Input: part model. Units: mm. Frame: model coordinates. Face numbers are marked on the shaded views. A direction names the side the tool comes from. Round coordinates to 2 decimals unless told otherwise and drop trailing zeros. Order: outer loops, then holes, each group sorted by start corner. A loop starts at its lowest first (then second) coordinate and runs counter-clockwise, first axis right, second up. Notation, with made-up numbers: (86.5, 65.25) -> (111.5, 65.25) arc R31 cw to (111.5, 94.25) -> close; hole circle Ø5 at (-17.5, 79.5). An arc over 180 degrees is marked (long way). Use a Markdown table: item, result.
from build123d import *

# Parameters (mm, degrees)
F0_R         = 1.8
F0_R_2       = 13.5
F0_W         = 20.1372796029
F0_H         = 5
F1_DEPTH     = 2
F2_W         = 3
F2_H         = 30
F3_DEPTH     = 27
F4_W         = 16.1372796029
F4_H         = 3
F5_DEPTH     = 25
F6_R         = 1.8
F6_W         = 4
F6_H         = 11
F7_DEPTH     = 25
F8_SIZE      = 25
F9_SIZE      = 14
F10_R        = 4.99999
F11_T1_DEPTH = 2
F11_T3_DEPTH = 32


# Not quite as in the source:
# - a fillet or chamfer that OpenCascade refuses, or shapes differently, is made with other operations: its cross-section is extruded or revolved along the edge and cut away or added
# - a fillet or chamfer is up to 0.001 mm smaller than in the source, because OpenCascade refuses the exact size


with BuildPart() as f1:
    # F0 (on Top) → F1 (new body)
    with BuildSketch(Plane.XY):
        Polygon((21.15, -21.15), (21.15, 21.15), (-21.15, 21.15), (-21.15, 3.85), (-21.15, -21.15), align=None)
        with Locations((-15.5, -15.5)):
            Circle(F0_R, mode=Mode.SUBTRACT)
        with Locations((15.5, -15.5)):
            Circle(F0_R, mode=Mode.SUBTRACT)
        with Locations((-15.5, 15.5)):
            Circle(F0_R, mode=Mode.SUBTRACT)
        Circle(F0_R_2, mode=Mode.SUBTRACT)
        with Locations((15.5, 15.5)):
            Circle(F0_R, mode=Mode.SUBTRACT)
        Polygon((-21.15, -21.15), (-21.15, 3.85), (-41.3, 3.85), (-41.3, -21.15), (-21.1627203971, -21.15), align=None)
        with Locations((-31.2313601986, -23.65)):
            Rectangle(F0_W, F0_H)
    extrude(amount=F1_DEPTH)

    # F2 (on Top) → F3 (join)
    with BuildSketch(Plane.XY):
        with Locations((-23.6627203971, -11.15)):
            Rectangle(F2_W, F2_H)
    extrude(amount=F3_DEPTH)

    # F4 (on face) → F5 (join)
    with BuildSketch(Plane.XY.offset(2)):
        with Locations((-33.2313601986, -24.65)):
            Rectangle(F4_W, F4_H)
    extrude(amount=F5_DEPTH)

    # F6 (on face) → F7 (cut)
    with BuildSketch(Plane(origin=(0, -23.15, 0), x_dir=(-1, 0, 0), z_dir=(0, 1, 0))):
        with Locations((35.5, 14.5)):
            Circle(F6_R)
        with Locations((35.5, 5.5)):
            Circle(F6_R)
        with Locations((35.5, 23.5)):
            Circle(F6_R)
        with Locations((28.2, 14.5)):
            Rectangle(F6_W, F6_H)
    extrude(amount=-F7_DEPTH, mode=Mode.SUBTRACT)

    # F8
    f8_edges = [f1.edges().sort_by_distance(p)[0] for p in [
        (-23.66272, 3.85, 27),
    ]]
    chamfer(f8_edges, length=F8_SIZE)

    # F9
    f9_edges = [f1.edges().sort_by_distance(p)[0] for p in [
        (-41.3, 3.85, 1),
    ]]
    chamfer(f9_edges, length=F9_SIZE)

    # F10 (radius 5 in the source; OpenCascade refuses exactly that, so slightly less here)
    f10_edges = [f1.edges().sort_by_distance(p)[0] for p in [
        (-41.3, -10.15, 1),
        (-27.3, 3.85, 1),
        (-21.16272, -26.15, 1),
        (-41.3, -24.65, 27),
    ]]
    fillet(f10_edges, radius=F10_R)

    # F11: fillet of radius 6 on 4 edges, made by hand

    # F11_s2 → F11_t1 (join)
    with BuildSketch(Plane.XY):
        with BuildLine():
            ThreePointArc((-26.1021461366, 3.7731598692), (-22.5517871308, 5.8265464621), (-21.15, 9.6809515277))
            Line((-21.15, 9.6809515277), (-20.55, 9.6809515277))
            Line((-20.55, 9.6809515277), (-20.55, 3.85))
            Line((-20.55, 3.85), (-21.15, 3.25))
            ThreePointArc((-21.15, 3.25), (-25.2289363303, 3.25), (-25.9973607503, 3.1823807033))
            Line((-25.9973607503, 3.1823807033), (-26.1021461366, 3.7731598692))
        make_face()
    extrude(amount=F11_T1_DEPTH)

    # F11_s4 → F11_t3 (cut)
    with BuildSketch(Plane.XY.offset(-15)):
        with BuildLine():
            ThreePointArc((21.15, -15.15), (19.3926406871, -19.3926406871), (15.15, -21.15))
            Line((15.15, -21.15), (21.15, -21.15))
            Line((21.15, -21.15), (21.15, -15.15))
        make_face()
        with BuildLine():
            ThreePointArc((15.15, 21.15), (19.3926406871, 19.3926406871), (21.15, 15.15))
            Line((21.15, 15.15), (21.15, 21.15))
            Line((21.15, 21.15), (15.15, 21.15))
        make_face()
        with BuildLine():
            ThreePointArc((-21.15, 15.15), (-19.3926406871, 19.3926406871), (-15.15, 21.15))
            Line((-15.15, 21.15), (-21.15, 21.15))
            Line((-21.15, 21.15), (-21.15, 15.15))
        make_face()
    extrude(amount=F11_T3_DEPTH, mode=Mode.SUBTRACT)


solid = f1.part
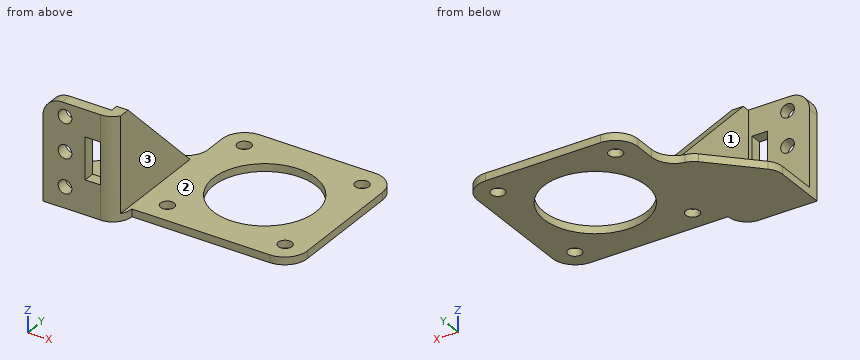
1) Ray query, probe 1 along Z at (x, y) = (-35.5, -25.05); probe 2 along Y at (x, z) = (-15.5, 0.9); probe 3 along Y at (x, z) = (15.5, 0.5). Return the intervals inside material, ascending.
Answer key:
| item | result |
|---|---|
| probe 1 | z = 0 to 3.7, 7.3 to 12.7, 16.3 to 21.7, 25.3 to 27 |
| probe 2 | y = -21.15 to -17.3, -13.7 to 13.7, 17.3 to 21.14 |
| probe 3 | y = -21.14 to -17.3, -13.7 to 13.7, 17.3 to 21.14 |
2) Set-up query: the marked faces 1, 2 and 3. Return all of +Z, -Z, +X, -X, +Y, -Y with unobstructed straight access to the full face (end or side cutting, diameter ignored); none if empty.
Answer key:
| item | result |
|---|---|
| face 1 | +Z, -X, +Y |
| face 2 | +Z, +Y |
| face 3 | +Z, +X, +Y, -Y |
3) Cut plane C-C on y = 0. Return loops of the section in (x, z), and give its area (4 significant figures).
Answer key:
| item | result |
|---|---|
| outline | (-31.15, 0) -> (-13.5, 0) -> (-13.5, 2) -> (-22.16, 2) -> (-22.16, 5.85) -> (-25.16, 5.85) -> (-25.16, 2) -> (-31.15, 2) -> close; (13.5, 0) -> (21.15, 0) -> (21.15, 2) -> (13.5, 2) -> close |
| area | 62.15 mm^2 |
4) Contact query for flat-ended pins moving along their axis: P1, Ø5, axis at x = -23.5, z = 18.5, coming from the -Y side; P2, Ø4, axis at x = -15.5, y = -15.5, coming from the +Z side; P3, Ø4, axis at y = -5.5, z = 13, coming from the -X side; P4, Ø24.5, axis at x = 0, y = 0, coming from the +Z side. Output: stop coordinate, or through.
Answer key:
| item | result |
|---|---|
| P1 | stops at y = -26.15 |
| P2 | stops at z = 2 |
| P3 | stops at x = -25.16 |
| P4 | passes through |
5) Cut plane D-D on z = 14.5. State how many separate pieces and enclosed holes the cut face has, and give its area (3 significant figures).
Answer key:
| item | result |
|---|---|
| separate pieces | 3 |
| enclosed holes | 0 |
| area | 75.7 mm^2 |
6) Cut plane A-A on z = 5.5. Return loops of the section in (x, y).
Answer key:
| item | result |
|---|---|
| outline | (-41.3, -26.15) -> (-37.3, -26.15) -> (-37.3, -23.15) -> (-41.3, -23.15) -> close; (-33.7, -26.15) -> (-26.16, -26.15) arc R5 ccw to (-22.16, -24.15) -> (-22.16, 0.35) -> (-25.16, 0.35) -> (-25.16, -23.15) -> (-33.7, -23.15) -> close |
7) Cut plane B-B on x = -35.5. Return loops of the section in (y, z), and give its area (3 significant figures).
Answer key:
| item | result |
|---|---|
| outline | (-26.15, 0) -> (-4.35, 0) -> (-4.35, 2) -> (-23.15, 2) -> (-23.15, 3.7) -> (-26.15, 3.7) -> close; (-26.15, 7.3) -> (-23.15, 7.3) -> (-23.15, 12.7) -> (-26.15, 12.7) -> close; (-26.15, 16.3) -> (-23.15, 16.3) -> (-23.15, 21.7) -> (-26.15, 21.7) -> close; (-26.15, 25.3) -> (-23.15, 25.3) -> (-23.15, 27) -> (-26.15, 27) -> close |
| area | 86.2 mm^2 |
